from build123d import *

# Parameters (mm, degrees)
F0_W     = 254
F0_H     = 127
F0_W_2   = 127
F0_H_2   = 88.9
F1_DEPTH = 127
F2_R     = 6.35
F3_R     = 31.75
F3_R_2   = 19.05
F4_DEPTH = 127
F5_R     = 6.35
F6_SIZE  = 3.175


with BuildPart() as f1:
    # F0 (on Top) → F1 (new body)
    with BuildSketch(Plane.XY):
        Rectangle(F0_W, F0_H)
        Rectangle(F0_W_2, F0_H_2, mode=Mode.SUBTRACT)
    extrude(amount=F1_DEPTH)

    # F2
    f2_edges = [f1.edges().sort_by_distance(p)[0] for p in [
        (127, 0, 127),
        (0, 63.5, 127),
        (-127, 0, 127),
        (0, -63.5, 127),
        (0, -44.45, 127),
        (-63.5, 0, 127),
        (0, 44.45, 127),
        (63.5, 0, 127),
        (127, 0, 0),
        (0, 63.5, 0),
        (-127, 0, 0),
        (0, -63.5, 0),
        (0, -44.45, 0),
        (-63.5, 0, 0),
        (0, 44.45, 0),
        (63.5, 0, 0),
        (-127, -63.5, 63.5),
        (127, -63.5, 63.5),
        (127, 63.5, 63.5),
        (-127, 63.5, 63.5),
    ]]
    fillet(f2_edges, radius=F2_R)

    # F3 (on face) → F4 (join)
    with BuildSketch(Plane.YZ.offset(127)):
        with Locations((0, 63.5)):
            Circle(F3_R)
        with Locations((0, 63.5)):
            Circle(F3_R_2, mode=Mode.SUBTRACT)
    extrude(amount=F4_DEPTH)

    # F5
    f5_edges = [f1.edges().sort_by_distance(p)[0] for p in [
        (127, -31.75, 63.5),
        (254, -31.75, 63.5),
    ]]
    fillet(f5_edges, radius=F5_R)

    # F6
    f6_edges = [f1.edges().sort_by_distance(p)[0] for p in [
        (254, -19.05, 63.5),
    ]]
    chamfer(f6_edges, length=F6_SIZE)


solid = f1.part
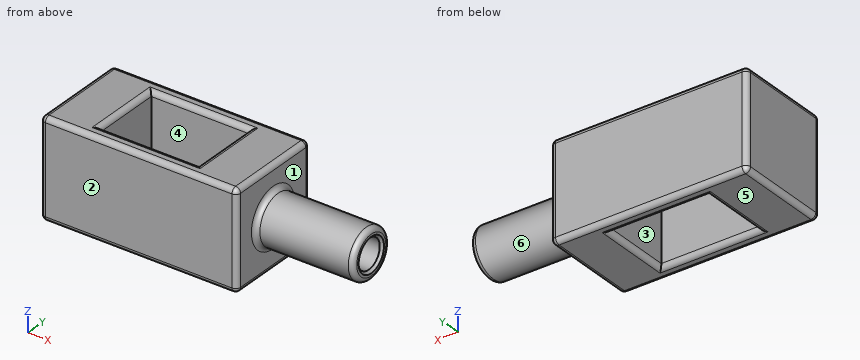
Check sheet for the modelled part. Datum: model origin and axes. Units: mm. Face numbers are marked on the shaded views. A direction names the side the tool comes from. Round coordinates to 2 decimals unless told otherwise and drop trailing zeros. Loops run counter-clockwise (first coordinate to the right, second up) from the corner with the lowest first, then second, coordinate; pieces in that order, holes last. Notation, with made-up numbers: (1, 80.5) -> (13, 80.5) arc R24 cw to (13, 92.5) -> close; hole circle Ø11 at (-34.5, -37.75). An arc over 180 degrees is marked (long way). Put each result on its own line as item: value. Start each with the question number.
1. Section check D-D (x = 165.5). Enter the section's corners in (y, z), plus the area to 3 significant figures.
2. Scan lines: probe 1 along Y at (x, z) = (58, 44); probe 2 along Y at (x, z) = (180, 63); probe 3 along Z at (x, y) = (207, 0). Record each from-to range of solid material in increasing order.
3. Section check C-C (z = 63.5). Enter the section's corners in (x, y) (3 decimals).
4. Section check B-B (x = 43). Enter the section's corners in (y, z), plus the area to 3 significant figures.
5. Draft check along Y on the marked faces 4, 5 and 6. Enter one of: +Y half, -Y half, draft (parallel to the pull), parting line (faces both ways), or undercut.
6. Gauge pin test, flat ends, axial feed: pin 1 (19 mm diameter, centred on y = 4.5, z = 71, fed in from +X); pin 2 (3 mm diameter, centred on y = -36.5, z = 71.5, fed in from +X). Record the tip position at first contact, or that the pin passes through.
7. Access from +Z, -Z, +X, -X, +Y, -Y to the whole of each face (thin tool, end or side, straight path). Record for the marked faces 1, 2 and 3.
Findings:
1. outline: circle Ø63.5 at (0, 63.5); hole circle Ø38.1 at (0, 63.5)
1. area: 2,030 mm^2
2. probe 1: y = -63.5 to -44.45, 44.45 to 63.5
2. probe 2: y = -31.75 to -19.04, 19.04 to 31.75
2. probe 3: z = 31.75 to 44.45, 82.55 to 95.25
3. outline: (-127, -57.15) arc R6.35 ccw to (-120.65, -63.5) -> (120.65, -63.5) arc R6.35 ccw to (127, -57.15) -> (127, -38.1) arc R6.35 cw to (133.35, -31.75) -> (247.65, -31.75) arc R6.35 ccw to (254, -25.4) -> (254, -22.225) -> (250.825, -19.05) -> (127, -19.05) -> (127, 19.05) -> (250.825, 19.05) -> (254, 22.225) -> (254, 25.4) arc R6.35 ccw to (247.65, 31.75) -> (133.35, 31.75) arc R6.35 cw to (127, 38.1) -> (127, 57.15) arc R6.35 ccw to (120.65, 63.5) -> (-120.65, 63.5) arc R6.35 ccw to (-127, 57.15) -> close; hole (-63.5, -44.45) -> (63.5, -44.45) -> (63.5, 44.45) -> (-63.5, 44.45) -> close
4. outline: (-63.5, 6.35) arc R6.35 ccw to (-57.15, 0) -> (-50.8, 0) arc R6.35 ccw to (-44.45, 6.35) -> (-44.45, 120.65) arc R6.35 ccw to (-50.8, 127) -> (-57.15, 127) arc R6.35 ccw to (-63.5, 120.65) -> close; (44.45, 6.35) arc R6.35 ccw to (50.8, 0) -> (57.15, 0) arc R6.35 ccw to (63.5, 6.35) -> (63.5, 120.65) arc R6.35 ccw to (57.15, 127) -> (50.8, 127) arc R6.35 ccw to (44.45, 120.65) -> close
4. area: 4,770 mm^2
5. face 4: undercut
5. face 5: draft
5. face 6: parting line
6. pin 1: stops at x = 127
6. pin 2: stops at x = 127.41
7. face 1: +X
7. face 2: +Z, -Z, +X, -X, -Y
7. face 3: +Z, -Z
